Model file for the job. Use its own axes, mm. Face numbers are marked on the shaded views. A direction names the side the tool comes from. Coordinates: 2 decimals unless noted, no trailing zeros. Order: outer loops, then holes, each group sorted by start corner. A loop starts at its lowest first (then second) coordinate and runs counter-clockwise, first axis right, second up. Notation, with made-up numbers: (63.5, 33.5) -> (73.5, 33.5) arc R29 ccw to (73.5, 68.5) -> close; hole circle Ø11 at (70, -33). An arc over 180 degrees is marked (long way). Use CSV: the item, a comma, the result in double quotes. Start each with the question number.
(1) Cut at C-C on z = 3.5. Write the cut outline in (x, y), plus the area to 3 significant figures.
(2) Pin check, flat tips, straight feed: pin 1 Ø7 at (x, y) = (-17, -20) entering from +Z; pin 2 Ø4 at (x, z) = (6, 13.5) entering from +Y; pin 3 Ø3.5 at (y, z) = (7, 17.5) entering from -X; pin 4 Ø2 at (x, y) = (-17, -20) entering from +Z. Stop position of each tip, or through.
(3) Cut at B-B on x = 0. Write the cut outline in (y, z).
(4) Pull direction X, two halves, no side cores. Call the marked faces 4, 5 and 6: pulls with the +X half, pulls with the -X half, needs draft (parallel to the pull), parting line crosses it, or undercut.
(5) Tool access for the marked faces 1, 2 and 3: list every direction of +Z, -Z, +X, -X, +Y, -Y with a clear straight run to the whole face (end or side of a thin tool).
(6) Probe L1, parallel to Y at x = -17, z = 2.2; L2, parallel to Y at x = -17, z = 5.45; L3, parallel to Z at x = -22, y = 24.5. List the from-to ranges inside material, lowest first.
(7) Cut at D-D on z = 8.5. Write the cut outline in (x, y), plus the area to 3 significant figures.
(8) Cut at A-A on y = 20. Write the cut outline in (x, z), plus the area to 3 significant figures.
```python
from build123d import *

# Parameters (mm, degrees)
F0_W     = 60
F0_H     = 60
F1_DEPTH = 7
F2_DEPTH = 20
F3_R     = 8.4497474683
F4_R     = 5
F5_R     = 1
F6_R     = 2.1
F7_DEPTH = 25
F6_R_2   = 3.75
F8_DEPTH = 2.7


# Not quite as in the source:
# - a feature names something its author has since deleted; it is built from what else it names


with BuildPart() as f1:
    # F0 (on Top) → F1 (new body)
    with BuildSketch(Plane.XY):
        Rectangle(F0_W, F0_H)
        with BuildLine():
            ThreePointArc((-16.7705098312, 10), (0, 22.5), (16.7705098312, 10))
            Line((16.7705098312, 10), (17.5, 10))
            Line((17.5, 10), (17.5, 5))
            ThreePointArc((17.5, 5), (0, -12.5), (-17.5, 5))
            Line((-17.5, 5), (-17.5, 10))
            Line((-17.5, 10), (-16.7705098312, 10))
        make_face(mode=Mode.SUBTRACT)
        with BuildLine():
            ThreePointArc((-12.5, 5), (0, -7.5), (12.5, 5))
            ThreePointArc((12.5, 5), (0, 17.5), (-12.5, 5))
        make_face()
        with BuildLine():
            ThreePointArc((-12.5, 5), (0, 17.5), (12.5, 5))
            Line((12.5, 5), (12.5, 10))
            Line((12.5, 10), (16.7705098312, 10))
            ThreePointArc((16.7705098312, 10), (0, 22.5), (-16.7705098312, 10))
            Line((-16.7705098312, 10), (-12.5, 10))
            Line((-12.5, 10), (-12.5, 5))
        make_face()
        with BuildLine():
            Line((12.5, 10), (12.5, 5))
            ThreePointArc((12.5, 5), (0, -7.5), (-12.5, 5))
            Line((-12.5, 5), (-12.5, 10))
            Line((-12.5, 10), (-16.7705098312, 10))
            ThreePointArc((-16.7705098312, 10), (-17.3166671454, 7.5264676876), (-17.5, 5))
            ThreePointArc((-17.5, 5), (0, -12.5), (17.5, 5))
            ThreePointArc((17.5, 5), (17.3166671454, 7.5264676876), (16.7705098312, 10))
            Line((16.7705098312, 10), (12.5, 10))
        make_face()
        with BuildLine():
            ThreePointArc((-17.5, 5), (-17.3166671454, 7.5264676876), (-16.7705098312, 10))
            Line((-16.7705098312, 10), (-17.5, 10))
            Line((-17.5, 10), (-17.5, 5))
        make_face()
        with BuildLine():
            Line((17.5, 10), (16.7705098312, 10))
            ThreePointArc((16.7705098312, 10), (17.3166671454, 7.5264676876), (17.5, 5))
            Line((17.5, 5), (17.5, 10))
        make_face()
    extrude(amount=F1_DEPTH)

    # F0 (on Top) → F2 (join)
    with BuildSketch(Plane.XY):
        with BuildLine():
            Line((12.5, 10), (12.5, 5))
            ThreePointArc((12.5, 5), (0, -7.5), (-12.5, 5))
            Line((-12.5, 5), (-12.5, 10))
            Line((-12.5, 10), (-16.7705098312, 10))
            ThreePointArc((-16.7705098312, 10), (-17.3166671454, 7.5264676876), (-17.5, 5))
            ThreePointArc((-17.5, 5), (0, -12.5), (17.5, 5))
            ThreePointArc((17.5, 5), (17.3166671454, 7.5264676876), (16.7705098312, 10))
            Line((16.7705098312, 10), (12.5, 10))
        make_face()
        with BuildLine():
            Line((17.5, 10), (16.7705098312, 10))
            ThreePointArc((16.7705098312, 10), (17.3166671454, 7.5264676876), (17.5, 5))
            Line((17.5, 5), (17.5, 10))
        make_face()
        with BuildLine():
            ThreePointArc((-17.5, 5), (-17.3166671454, 7.5264676876), (-16.7705098312, 10))
            Line((-16.7705098312, 10), (-17.5, 10))
            Line((-17.5, 10), (-17.5, 5))
        make_face()
    extrude(amount=F2_DEPTH)

    # F3
    f3_edges = [f1.edges().sort_by_distance(p)[0] for p in [
        (0, -12.5, 7),
        (-17.5, 7.5, 7),
        (17.5, 7.5, 7),
    ]]
    fillet(f3_edges, radius=F3_R)

    # F4
    f4_edges = [f1.edges().sort_by_distance(p)[0] for p in [
        (30, -30, 3.5),
        (-30, -30, 3.5),
        (-30, 30, 3.5),
        (30, 30, 3.5),
    ]]
    fillet(f4_edges, radius=F4_R)

    # F5
    f5_edges = [f1.edges().sort_by_distance(p)[0] for p in [
        (-30, 0, 7),
        (-28.535534, 28.535534, 7),
        (0, 30, 7),
        (30, 0, 7),
        (28.535534, 28.535534, 7),
        (0, -30, 7),
        (-28.535534, -28.535534, 7),
        (28.535534, -28.535534, 7),
    ]]
    fillet(f5_edges, radius=F5_R)

    # F6 (on face) → F7 (cut)
    with BuildSketch(Plane.XY.offset(7)):
        with Locations((-17, 20)):
            Circle(F6_R)
        with Locations((17, 20)):
            Circle(F6_R)
        with Locations((-17, -20)):
            Circle(F6_R)
        with Locations((17, -20)):
            Circle(F6_R)
    extrude(amount=-F7_DEPTH, mode=Mode.SUBTRACT)

    # F6 (on face) → F8 (cut)
    with BuildSketch(Plane.XY.offset(7)):
        with Locations((-17, 20)):
            Circle(F6_R_2)
        with Locations((-17, 20)):
            Circle(F6_R, mode=Mode.SUBTRACT)
        with Locations((17, 20)):
            Circle(F6_R_2)
        with Locations((17, 20)):
            Circle(F6_R, mode=Mode.SUBTRACT)
        with Locations((-17, -20)):
            Circle(F6_R_2)
        with Locations((-17, -20)):
            Circle(F6_R, mode=Mode.SUBTRACT)
        with Locations((17, -20)):
            Circle(F6_R_2)
        with Locations((17, -20)):
            Circle(F6_R, mode=Mode.SUBTRACT)
    extrude(amount=-F8_DEPTH, mode=Mode.SUBTRACT)


solid = f1.part
```
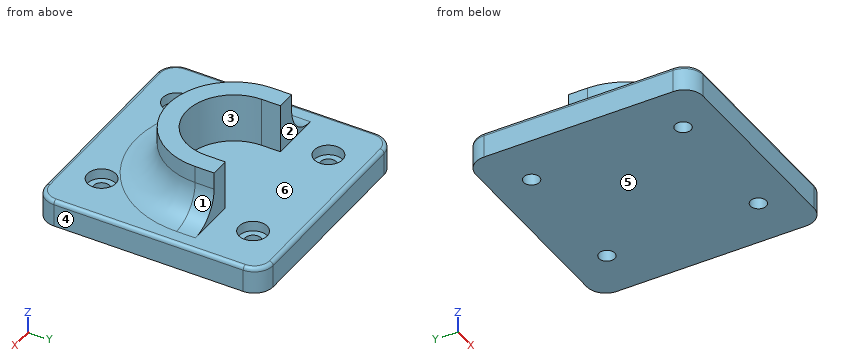
Outcome:
1,outline,"(-30, -25) arc R5 ccw to (-25, -30) -> (25, -30) arc R5 ccw to (30, -25) -> (30, 25) arc R5 ccw to (25, 30) -> (-25, 30) arc R5 ccw to (-30, 25) -> close; hole circle Ø4.2 at (-17, -20); hole circle Ø4.2 at (-17, 20); hole circle Ø4.2 at (17, -20); hole circle Ø4.2 at (17, 20)"
1,area,"3,520 mm2"
2,pin 1,"z = 4.3"
2,pin 2,"y = -4.6"
2,pin 3,"x = -17.5"
2,pin 4,"through"
3,outline,"(-30, 0) -> (30, 0) -> (30, 6) arc R1 ccw to (29, 7) -> (-7.5, 7) -> (-7.5, 20) -> (-12.5, 20) -> (-12.5, 15.45) arc R8.45 cw to (-20.95, 7) -> (-29, 7) arc R1 ccw to (-30, 6) -> close"
4,face 4,"pulls with the +X half"
4,face 5,"needs draft"
4,face 6,"undercut"
5,face 1,"+Z, +X, +Y, -Y"
5,face 2,"+Z, +X, -X, +Y"
5,face 3,"+Z, +Y"
6,L1,"-30 to -22.1, -17.9 to 17.9, 22.1 to 30"
6,L2,"-30 to -23.75, -16.25 to 16.25, 23.75 to 30"
6,L3,"0 to 7"
7,outline,"(-21.14, 5) arc R21.14 ccw to (21.14, 5) -> (21.14, 10) -> (12.5, 10) -> (12.5, 5) arc R12.5 cw to (-12.5, 5) -> (-12.5, 10) -> (-21.14, 10) -> close"
7,area,"543 mm2"
8,outline,"(-30, 0) -> (-19.1, 0) -> (-19.1, 4.3) -> (-20.75, 4.3) -> (-20.75, 7) -> (-29, 7) arc R1 ccw to (-30, 6) -> close; (-14.9, 0) -> (14.9, 0) -> (14.9, 4.3) -> (13.25, 4.3) -> (13.25, 7) -> (-13.25, 7) -> (-13.25, 4.3) -> (-14.9, 4.3) -> close; (19.1, 0) -> (30, 0) -> (30, 6) arc R1 ccw to (29, 7) -> (20.75, 7) -> (20.75, 4.3) -> (19.1, 4.3) -> close"
8,area,"343 mm2"
